```python
from build123d import *

# Parameters (mm, degrees)
SKETCH1_R            = 7.518485851
BOSS_EXTRUDE1_DEPTH  = 30
SKETCH7_R            = 5.956950852
CUT_EXTRUDE1_DEPTH   = 60
SKETCH8_W            = 2
SKETCH8_H            = 7.5
BOSS_EXTRUDE4_DEPTH  = 5.5
CIRPATTERN7_COUNT    = 6
SKETCH13_W           = 13.226989642
SKETCH13_H           = 2.75
BOSS_EXTRUDE6_DEPTH  = 5.5
BOSS_EXTRUDE7_DEPTH  = 5.516040115
CIRPATTERN10_COUNT   = 3
BOSS_EXTRUDE8_DEPTH  = 5.5
BOSS_EXTRUDE11_DEPTH = 5.5
BOSS_EXTRUDE12_DEPTH = 5.5
BOSS_EXTRUDE13_DEPTH = 5.5
SKETCH30_W           = 1.493482136
SKETCH30_H           = 1.466135263
BOSS_EXTRUDE15_DEPTH = 2.5
CIRPATTERN11_COUNT   = 4


with BuildPart() as part:
    # Sketch1 → Boss-Extrude1 (new body)
    with BuildSketch(Plane(origin=(0, 0, 0), x_dir=(1, 0, 0), z_dir=(0, 1, 0))):
        with Locations(Location((0, 0, 0), (0, 0, 270))):
            Circle(SKETCH1_R)
    extrude(amount=BOSS_EXTRUDE1_DEPTH)

    # Sketch7 → Cut-Extrude1 (cut)
    with BuildSketch(Plane(origin=(0, 30, 0), x_dir=(1, 0, 0), z_dir=(0, 1, 0))):
        with Locations(Location((0, 0, 0), (0, 0, 270))):
            Circle(SKETCH7_R)
    extrude(amount=-CUT_EXTRUDE1_DEPTH, mode=Mode.SUBTRACT)

    # Sketch8 → Boss-Extrude4 (add)
    with BuildSketch(Plane(origin=(0, 30, 0), x_dir=(1, 0, 0), z_dir=(0, 1, 0))):
        with Locations((0.055499062, 11.208924015)):
            Rectangle(SKETCH8_W, SKETCH8_H)
    boss_extrude4 = extrude(amount=-BOSS_EXTRUDE4_DEPTH)

    # CirPattern7: Boss-Extrude4 ×6 about axis
    cirpattern7_axis = Axis((0, 0, 0), (0, 1, 0))
    for i in range(1, CIRPATTERN7_COUNT):
        add(boss_extrude4.rotate(cirpattern7_axis, i * 360 / CIRPATTERN7_COUNT))

    # Sketch13 → Revolve1 (revolve)
    with BuildSketch(Plane(origin=(6.678494764, 0, 11.680402876), x_dir=(-0.8681157278989303, 0, 0.4963618468159196), z_dir=(-0.49636184681591955, 0, -0.8681157278989302))):
        with Locations((-0.00839179, 28.625)):
            Rectangle(SKETCH13_W, SKETCH13_H)
    revolve1 = revolve(axis=Axis((0.944500938, 27.25, 14.958924015), (0.8681157278989303, 0, -0.4963618468159195)))

    # Sketch15 → Boss-Extrude6 (add)
    with BuildSketch(Plane(origin=(0, 30, 0), x_dir=(1, 0, 0), z_dir=(0, 1, 0))):
        with BuildLine():
            Line((2.309496017, -17.346242267), (0.944500938, -14.958924015))
            Line((0.944500938, -14.958924015), (-1.055499062, -14.958924015))
            add(Edge.make_bspline(
                [(-1.055499062, -14.958924015), (-0.826479447, -16.658649969), (0.315527094, -17.640821071), (2.309496017, -17.346242267)],
                knots=[0, 0, 0, 0, 1, 1, 1, 1], degree=3))
        make_face()
    extrude(amount=-BOSS_EXTRUDE6_DEPTH)

    # Sketch20 → Boss-Extrude7 (add)
    with BuildSketch(Plane(origin=(0, 30, 0), x_dir=(1, 0, 0), z_dir=(0, 1, 0))):
        with BuildLine():
            Line((13.792053758, -10.78086926), (12.42705868, -8.393551008))
            Line((12.42705868, -8.393551008), (13.42705868, -6.661500201))
            add(Edge.make_bspline(
                [(13.42705868, -6.661500201), (14.923928961, -8.195328029), (14.840637873, -9.355950273), (13.792053758, -10.78086926)],
                knots=[0, 0, 0, 0, 1, 1, 1, 1], degree=3))
        make_face()
    extrude(amount=-BOSS_EXTRUDE7_DEPTH)

    # CirPattern10: Revolve1 ×3 about axis
    cirpattern10_axis = Axis((0, -30, 0), (0, 1, 0))
    for i in range(1, CIRPATTERN10_COUNT):
        add(revolve1.rotate(cirpattern10_axis, i * 360 / CIRPATTERN10_COUNT))

    # Sketch21 → Boss-Extrude8 (add)
    with BuildSketch(Plane(origin=(0, 30, 0), x_dir=(1, 0, 0), z_dir=(0, 1, 0))):
        with BuildLine():
            Line((-16.232533533, -6.553834295), (-13.482557741, -6.565373007))
            Line((-13.482557741, -6.565373007), (-12.482557741, -8.297423814))
            add(Edge.make_bspline(
                [(-12.482557741, -8.297423814), (-15.604680205, -9.03295077), (-16.232533533, -6.553834295)],
                knots=[0, 0, 0, 1, 1, 1], degree=2))
        make_face()
    extrude(amount=-BOSS_EXTRUDE8_DEPTH)

    # Sketch24 → Boss-Extrude11 (add)
    with BuildSketch(Plane(origin=(0, 30, 0), x_dir=(1, 0, 0), z_dir=(0, 1, 0))):
        with BuildLine():
            Line((-13.42705868, 6.661500201), (-16.177034472, 6.673038913))
            add(Edge.make_bspline(
                [(-12.42705868, 8.393551008), (-14.838115801, 8.181475497), (-16.177034472, 6.673038913)],
                knots=[0, 0, 0, 1, 1, 1], degree=2))
            Line((-12.42705868, 8.393551008), (-13.42705868, 6.661500201))
        make_face()
    extrude(amount=-BOSS_EXTRUDE11_DEPTH)

    # Sketch26 → Boss-Extrude12 (add)
    with BuildSketch(Plane(origin=(0, 30, 0), x_dir=(1, 0, 0), z_dir=(0, 1, 0))):
        with BuildLine():
            Line((13.867538455, 10.673203354), (12.482557741, 8.297423814))
            Line((12.482557741, 8.297423814), (13.482557741, 6.565373007))
            add(Edge.make_bspline(
                [(13.482557741, 6.565373007), (15.18756028, 8.443349852), (13.867538455, 10.673203354)],
                knots=[0, 0, 0, 1, 1, 1], degree=2))
        make_face()
    extrude(amount=-BOSS_EXTRUDE12_DEPTH)

    # Sketch27 → Boss-Extrude13 (add)
    with BuildSketch(Plane(origin=(0, 30, 0), x_dir=(1, 0, 0), z_dir=(0, 1, 0))):
        with BuildLine():
            Line((-0.944500938, 14.958924015), (1.055499062, 14.958924015))
            Line((1.055499062, 14.958924015), (2.440479775, 17.334703555))
            add(Edge.make_bspline(
                [(-0.944500938, 14.958924015), (-0.189537041, 17.173381249), (2.440479775, 17.334703555)],
                knots=[0, 0, 0, 1, 1, 1], degree=2))
        make_face()
    extrude(amount=-BOSS_EXTRUDE13_DEPTH)

    # Sketch30 → Boss-Extrude15 (add)
    with BuildSketch(Plane(origin=(0, 0, 0), x_dir=(-1, 0, 0), z_dir=(0, -1, 0))):
        with Locations((0, -6.69246192)):
            Rectangle(SKETCH30_W, SKETCH30_H)
    boss_extrude15 = extrude(amount=BOSS_EXTRUDE15_DEPTH)

    # CirPattern11: Boss-Extrude15 ×4 about axis
    cirpattern11_axis = Axis((0, 0, 0), (0, 1, 0))
    for i in range(1, CIRPATTERN11_COUNT):
        add(boss_extrude15.rotate(cirpattern11_axis, i * 360 / CIRPATTERN11_COUNT))


solid = part.part
```
Design review of the part built by this model. Coordinates are the model's own, in mm. A direction names the side the tool comes from. Give positions to 0.01 mm unless a question says otherwise; leave off trailing zeros. Loops run counter-clockwise (first coordinate to the right, second up) from the corner with the lowest first, then second, coordinate; pieces in that order, holes last. Notation, with made-up numbers: M 19,-26 L 52,-26 A27 cw 52,2 Z; hole C -18.5,38.25 d4. An arc over 180 degrees is marked long. Return JSON: item names as keys, results as strings. Group by question number.
Item 1: We need section B-B (x = 9). Give the number of separate pieces and of enclosed holes in the cut face, and give its area (3 significant figures).
Item 2: Mouldability with a two-part tool opening along X and no side actions: class faces 4 (the flat face through (10.189, 27.288, -4.664)), 5 (the flat face through (0.945, 27, 9)), 6 (the flat face through (-5.959, -1, 0)), 7 (the flat face through (11, 24.5, -6)) as released by +X, released by -X, zero draft, split by the parting line, or undercut.
Item 3: For probe 1 along X at (y, z) = (15.75, 0); probe 2 along Z at (x, y) = (3.5, 25.5); probe 3 along X at (y, z) = (27.5, -4.5), list the stretches that pass through material, from the lowest coordinate up.
Item 4: We need section A-A (y = 23). Give the boundary of the cut face in (x, z).
Item 5: Tool access review of faces 1 (the flat face through (0, -1, -5.959)), 2 (the flat face through (7, -1, 0.747)), 3 (the flat face through (0, -1, -7.426)): name each direction out of +Z, -Z, +X, -X, +Y, -Y from which nothing blocks a thin tool from reaching the whole face with its end or side.
Item 6: Insertion check: pin 1 Ø1.6 at (x, y) = (6.5, -1.5) entering from -Z; pin 2 Ø5 at (y, z) = (9.5, 4) entering from +X; pin 3 Ø1.6 at (x, y) = (-0.5, -2) entering from -Z; pin 4 Ø10 at (y, z) = (26.5, 7.5) entering from -X. Each pin has a flat end and moves straight along its axis. Give the tip position at first contact, or say it passes through.
Output:
{
 "1": {"separate pieces": "4", "enclosed holes": "0", "area": "80.3 mm^2"},
 "2": {"face 4": "released by +X", "face 5": "undercut", "face 6": "undercut", "face 7": "zero draft"},
 "3": {"probe 1": "x = -7.52 to -5.96, 5.96 to 7.52", "probe 2": "z = -15.99 to -11.08, -6.65 to -4.82, 4.82 to 6.65, 11.05 to 15.94", "probe 3": "x = -16.17 to -10.7, -9.68 to -3.9, 3.9 to 9.91"},
 "4": {"outline": "C 0,0 d15.04; hole C 0,0 d11.91"},
 "5": {"face 1": "+X, -X, -Y", "face 2": "+Z, +X, -X, -Y", "face 3": "-Z, +X, -X, -Y"},
 "6": {"pin 1": "stops at z = -0.75", "pin 2": "stops at x = 7.37", "pin 3": "stops at z = -7.43", "pin 4": "stops at x = -16.23"}
}
